Input: part model. Units: mm. Frame: model coordinates. Face numbers are marked on the shaded views. Give positions to 0.01 mm unless a question says otherwise; leave off trailing zeros. Order: outer loops, then holes, each group sorted by start corner. A loop starts at its lowest first (then second) coordinate and runs counter-clockwise, first axis right, second up. Notation, with made-up numbers: (9, 44.25) -> (23, 44.25) arc R31 cw to (23, 75.25) -> close; hole circle Ø4 at (52, -36.5). An arc over 180 degrees is marked (long way). Use a Markdown table: item, result. Add a question column.
from build123d import *

# Parameters (mm, degrees)
F0_R     = 5
F1_DEPTH = 76.1
F2_R     = 5
F3_W     = 10
F3_H     = 1
F4_DEPTH = 33.75
F5_R     = 2.75
F6_DEPTH = 12.5
F8_D     = 8.4
F8_DEPTH = 20
F8_TIP   = 2.5236145999


with BuildPart() as f1:
    # F0 (on Right) → F1 (new body)
    with BuildSketch(Plane.YZ):
        Circle(F0_R)
    extrude(amount=F1_DEPTH)

    # F2
    f2_edges = [f1.edges().sort_by_distance(p)[0] for p in [
        (0, -5, 0),
    ]]
    fillet(f2_edges, radius=F2_R)

    # F3 (on Right) → F4 (cut)
    with BuildSketch(Plane.YZ):
        Rectangle(F3_W, F3_H)
    extrude(amount=F4_DEPTH, mode=Mode.SUBTRACT)

    # F5 (on Front) → F6 (cut, symmetric)
    with BuildSketch(Plane.XZ):
        with Locations((33.75, 0)):
            Circle(F5_R)
    extrude(amount=F6_DEPTH, both=True, mode=Mode.SUBTRACT)

    # F8
    with Locations(Plane.YZ.offset(76.1)):
        with Locations((0, 0)):
            Hole(F8_D / 2, depth=F8_DEPTH)
            with Locations((0, 0, -(F8_DEPTH + F8_TIP / 2))):  # 118° drill point
                Cone(0, F8_D / 2, F8_TIP, mode=Mode.SUBTRACT)


solid = f1.part
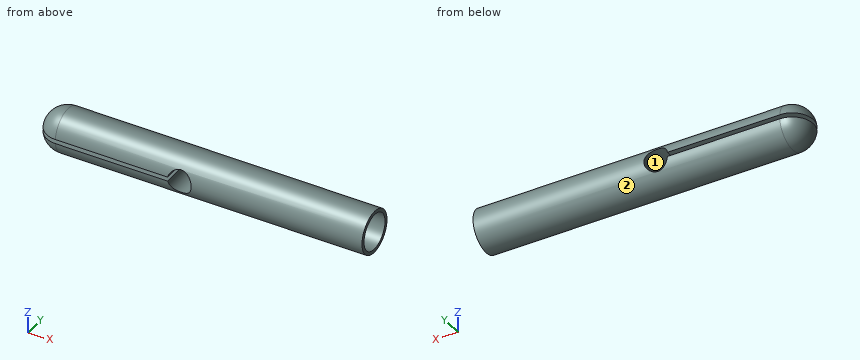
Q1. Section query B-B (x = 67). Return loops of the section in (y, z).
Q2. Ray query, line 1 (Y direction, x = 63, z = 0); line 2 (Z direction, x = 33.75, y = -0.5). Return the intervals inside material, ascending.
Q3. Draft query along Z for the marked faces 1 and 2. Return one class per face: +Z half, -Z half, draft (parallel to the pull), parting line (faces both ways), or undercut.
Q4. First-contact query: pin 1 (6 mm diameter, centred on x = 47.5, y = -3.5, fed in from -Z); pin 2 (1 mm diameter, centred on x = 44.5, z = 2.5, fed in from +Y); pin 3 (1 mm diameter, centred on y = -2.5, z = 1, fed in from -X). Flat tips, straight axial feed; report the tip coordinate or a pass-through.
Q5. Section query C-C (x = 52). Return loops of the section in (y, z), plus the area to 3 significant figures.
Solution:
| question | item | result |
|---|---|---|
| 1 | outline | circle Ø10 at (0, 0); hole circle Ø8.4 at (0, 0) |
| 2 | line 1 | y = -5 to -4.2, 4.2 to 5 |
| 2 | line 2 | z = -4.97 to -2.75, 2.75 to 4.97 |
| 3 | face 1 | undercut |
| 3 | face 2 | parting line |
| 4 | pin 1 | stops at z = -4.97 |
| 4 | pin 2 | stops at y = 4.58 |
| 4 | pin 3 | stops at x = 0.51 |
| 5 | outline | circle Ø10 at (0, 0) |
| 5 | area | 78.5 mm² |
